Input: part model. Units: mm. Frame: model coordinates. A direction names the side the tool comes from. Give positions to 0.01 mm unless a question says otherwise; leave off trailing zeros. Loops run counter-clockwise (first coordinate to the right, second up) from the corner with the lowest first, then second, coordinate; pieces in that order, holes last. Notation, with made-up numbers: M 79,13 L 83,13 A23 ccw 83,48 Z; hole C 2,-35.5 d9. An arc over 180 degrees is marked long. One line per item, written item: value. Start each with the question number.
(1) Ray query, line 1 along X through (y, z) = (-5.95, 23.75); line 2 along X through (y, z) = (7.5, 19); line 3 along Y through (x, z) = (-6.5, 1). Return the intervals inside material, ascending. Write a range as from..to.
(2) Pull-direction query (Z, two-part tool) for faces 1 (the cylindrical face through (-13.076, 12.342, 13.616)), 2 (the cylindrical face through (2.13, -5.87, 4.68)), 3 (the flat face through (6.52, 1.45, 3.36)); classes: released by +Z, released by -Z, zero draft, split by the parting line, or undercut.
(3) Section C-C on y = -3. Output: boundary loops of the cut face in (x, z).
(4) Pin query (flat end, axial travel): P1, Ø12, axis at x = -1.5, z = 24, coming from the +Y side. Return the tip coordinate at first contact, or that it passes through.
(5) Access query for faces 4 (the flat face through (5.833, 2, 13)), 5 (the flat face through (7.233, 1, 13)). Directions: +Z, -Z, +X, -X, +Y, -Y. A direction counts if a zero-diameter tool reaches every point of the face in a straight line with its end or side. Return the directions, or none.
(6) Section D-D on z = 23.75. Output: boundary loops of the cut face in (x, y).
(7) Section A-A on z = 13.5. Output: boundary loops of the cut face in (x, y), plus the area to 3 significant figures.
(8) Section B-B on x = -8.5. Output: boundary loops of the cut face in (y, z), plus the area to 3 significant figures.
Autodesk Inventor part; units mm, degrees
ref_plane "YZ Plane" through (0, 0, 0) normal (1, 0, 0) x (0, 1, 0)
ref_plane "XZ Plane" through (0, 0, 0) normal (0, 1, 0) x (-1, 0, 0)
ref_plane "XY Plane" through (0, 0, 0) normal (0, 0, 1) x (1, 0, 0)
sketch "Szkic1" plane through (0, 0, 0) normal (0, 0, 1) x (1, 0, 0)
  line L0 (-13.7667, 13.4433) -> (-13.7667, -6.5567)
  line L1 (-13.7667, -6.5567) -> (7.2333, -6.5567)
  line L2 (7.2333, -6.5567) -> (7.2333, 13.4433)
  line L3 (7.2333, 13.4433) -> (5.8333, 13.4433)
  line L4 (-13.7667, 13.4433) -> (-12.3667, 13.4433)
  line L5 (-12.3667, -5.1567) -> (5.8333, -5.1567)
  line L6 (5.8333, -5.1567) -> (5.8333, 13.4433)
  line L7 (-12.3667, 13.4433) -> (-12.3667, -5.1567)
  point P0 (0, 0)
  dimension "d0" = 21
  dimension "d1" = 20
  dimension "d2" = 1.4
  dimension "d3" = 1.4
  dimension "d4" = 1.4
extrude "Wyciągnięcie proste1" add sketch "Szkic1" along normal blind 27
sketch "Szkic2" plane through (-13.7667, -6.5567, 0) normal (-1, 0, 0) x (0, 0, 1)
  line L0 (0, 20) -> (0, 0)
  line L1 (0, 0) -> (27, 0)
  line L2 (27, 20) -> (27, 0)
  line L3 (0, 20) -> (27, 20)
  line L4 (0, 1.4) -> (27, 1.4)
  arc A0 (20.1851, 14.7999) -> (6.8149, 14.7999) centre (13.5, 11.4) ccw
  line L5 (27, 1.4) -> (27, 20)
  line L6 (27, 1.4) -> (20.1851, 14.7999)
  line L7 (0, 1.4) -> (0, 20)
  line L8 (0, 1.4) -> (6.8149, 14.7999)
  line L9 (6.8149, 14.7999) -> (9.4595, 20)
  line L10 (20.1851, 14.7999) -> (17.5405, 20)
  point P0 (0, 6.5567)
  dimension "d7" = 27
  dimension "d8" = 13.5
  dimension "d9" = 10
  dimension "d10" = 15
extrude "Wyciągnięcie proste2" cut sketch "Szkic2" against normal through all contours L3 L9 L8 L0 | L3 L10 A0 L9 | L6 L10 L3 L2
hole "Otwór1" at (-13.7667, 4.8433, 13.5) direction (1, 0, 0) diameter 4 end through all
sketch "Szkic3" plane through (-12.3667, -5.1567, 0) normal (0, 1, 0) x (1, 0, 0)
  line L0 (18.2, 0) -> (0, 0)
  line L1 (0, 0) -> (0, -27)
  line L2 (18.2, -27) -> (0, -27)
  line L3 (18.2, 0) -> (18.2, -27)
  line L4 (18.2, -20.5) -> (0, -20.5)
  line L5 (18.2, -6.5) -> (0, -6.5)
  point P0 (12.3667, 0)
  point P1 (14.95, -23.75)
  point P2 (3.25, -23.75)
  point P3 (14.95, -3.25)
  point P4 (3.25, -3.25)
  dimension "d20" = 14
  dimension "d21" = 27
  dimension "d22" = 6.5
  dimension "d23" = 3.25
  dimension "d24" = 3.25
  dimension "d25" = 3.25
  dimension "d26" = 3.25
  dimension "d27" = 3.25
  dimension "d28" = 3.25
  dimension "d29" = 3.25
  dimension "d30" = 3.25
hole "Otwór2" at (2.5833, -5.1567, 23.75) at (-9.1167, -5.1567, 23.75) at (2.5833, -5.1567, 3.25) at (-9.1167, -5.1567, 3.25) direction (0, -1, 0) diameter 3 end through all
equation "\"d22\" = -0.5 * d20 + 0.5 * d21"
properties part number "CNCM_Y_Axis_Tensioning_System_C_Sec_Idler"
Output values:
1. line 1: x = -13.77..-10.62, -7.62..1.08, 4.08..7.23
1. line 2: x = -13.77..-12.37, 5.83..7.23
1. line 3: y = -6.56..-5.16
2. face 1: split by the parting line
2. face 2: undercut
2. face 3: released by -Z
3. outline: M -13.77,1.1 L -12.37,1.1 L -12.37,25.9 L -13.77,25.9 Z; M 5.83,1.1 L 7.23,1.1 L 7.23,25.9 L 5.83,25.9 Z
4. P1: stops at y = -5.16
5. face 4: +Z, -Z, +Y
5. face 5: +Z, -Z, +X, +Y, -Y
6. outline: M -13.77,-6.56 L -10.62,-6.56 L -10.62,-5.16 L -12.37,-5.16 L -12.37,1.23 L -13.77,1.23 Z; M -7.62,-6.56 L 1.08,-6.56 L 1.08,-5.16 L -7.62,-5.16 Z; M 4.08,-6.56 L 7.23,-6.56 L 7.23,1.23 L 5.83,1.23 L 5.83,-5.16 L 4.08,-5.16 Z
7. outline: M -13.77,-6.56 L 7.23,-6.56 L 7.23,2.84 L 5.83,2.84 L 5.83,-5.16 L -12.37,-5.16 L -12.37,2.84 L -13.77,2.84 Z; M -13.77,6.84 L -12.37,6.84 L -12.37,12.34 L -13.77,12.34 Z; M 5.83,6.84 L 7.23,6.84 L 7.23,12.34 L 5.83,12.34 Z
7. area: 67.2 mm²
8. outline: M -6.56,0 L -5.16,0 L -5.16,1.88 L -6.56,1.88 Z; M -6.56,4.62 L -5.16,4.62 L -5.16,22.38 L -6.56,22.38 Z; M -6.56,25.12 L -5.16,25.12 L -5.16,27 L -6.56,27 Z
8. area: 30.1 mm²
